Input: part model. Units: mm. Frame: model coordinates. Face numbers are marked on the shaded views. A direction names the side the tool comes from. Give positions to 0.01 mm unless a question says otherwise; leave off trailing zeros. Write each loop counter-clockwise with the first axis right and the second up, starting at its lowest first coordinate (ties: lowest second). Pieces come first, ordered by that corner, then holes. Notation, with made-up numbers: (-35, -23.75) - (5, -23.75) arc R20 ccw to (5, -0.75) - close; hole circle Ø4 at (17.5, 79). An arc over 180 degrees is marked (long way). Answer as CSV lines item,"result".
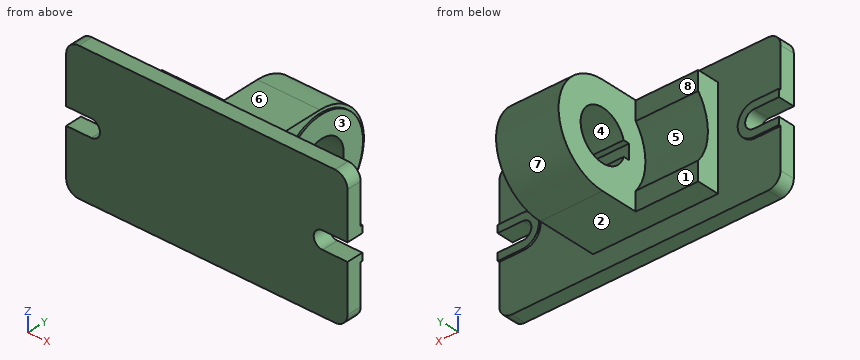
```python
from build123d import *

# Parameters (mm, degrees)
EXTRUDE_1_DEPTH     = 6
EXTRUDE_2_DEPTH     = 1.5
EXTRUDE_START       = -100
EXTRUDE_3_DEPTH     = 25
SKETCH_4_R          = 37.5
EXTRUDE_4_DEPTH     = 1.5
SKETCH_5_R          = 20
SKETCH_5_W          = 12
SKETCH_5_H          = 8
CUT_EXTRUDE_1_DEPTH = 187.58309141
SKETCH_6_W          = 50
SKETCH_6_H          = 80
EXTRUDE_5_DEPTH     = 1.5
SKETCH_7_W          = 15
SKETCH_7_H          = 16.5
EXTRUDE_6_DEPTH     = 50


with BuildPart() as part:
    # 草图1 → 凸台-拉伸1 (new, symmetric)
    with BuildSketch(Plane(origin=(0, 0, 0), x_dir=(1, 0, 0), z_dir=(0, 1, 0))):
        with BuildLine():
            ThreePointArc((-112.5, -45), (-109.571067812, -52.071067812), (-102.5, -55))
            Line((-102.5, -55), (102.5, -55))
            ThreePointArc((102.5, -55), (109.571067812, -52.071067812), (112.5, -45))
            Line((112.5, -45), (112.5, -7))
            Line((112.5, -7), (92.5, -7))
            ThreePointArc((92.5, -7), (85.5, 0), (92.5, 7))
            Line((92.5, 7), (112.5, 7))
            Line((112.5, 7), (112.5, 45))
            ThreePointArc((112.5, 45), (109.571067812, 52.071067812), (102.5, 55))
            Line((102.5, 55), (-102.5, 55))
            ThreePointArc((-102.5, 55), (-109.571067812, 52.071067812), (-112.5, 45))
            Line((-112.5, 45), (-112.5, 7))
            Line((-112.5, 7), (-92.5, 7))
            ThreePointArc((-92.5, 7), (-85.5, 0), (-92.5, -7))
            Line((-92.5, -7), (-112.5, -7))
            Line((-112.5, -7), (-112.5, -45))
        make_face()
    extrude(amount=EXTRUDE_1_DEPTH, both=True)

    # 草图2 → 凸台-拉伸2 (add, symmetric)
    with BuildSketch(Plane(origin=(0, 6, 0), x_dir=(1, 0, 0), z_dir=(0, 1, 0))):
        with BuildLine():
            Line((-92.5, 13), (-112.5, 13))
            Line((-112.5, 13), (-112.5, 7))
            Line((-112.5, 7), (-92.5, 7))
            ThreePointArc((-92.5, 7), (-85.5, 0), (-92.5, -7))
            Line((-92.5, -7), (-112.5, -7))
            Line((-112.5, -7), (-112.5, -13))
            Line((-112.5, -13), (-92.5, -13))
            ThreePointArc((-92.5, -13), (-79.5, 0), (-92.5, 13))
        make_face()
        with BuildLine():
            Line((112.5, 7), (112.5, 13))
            Line((112.5, 13), (92.5, 13))
            ThreePointArc((92.5, 13), (79.5, 0), (92.5, -13))
            Line((92.5, -13), (112.5, -13))
            Line((112.5, -13), (112.5, -7))
            Line((112.5, -7), (92.5, -7))
            ThreePointArc((92.5, -7), (85.5, 0), (92.5, 7))
            Line((92.5, 7), (112.5, 7))
        make_face()
    extrude(amount=EXTRUDE_2_DEPTH, both=True)

    # 草图3 → 凸台-拉伸3 (add, symmetric)
    with BuildSketch(Plane(origin=(112.5, 0, 0), x_dir=(0, 0, -1), z_dir=(1, 0, 0)).offset(EXTRUDE_START)):
        with BuildLine():
            Line((-40, 6), (40, 6))
            Line((40, 6), (40, 54))
            ThreePointArc((40, 54), (0, 94), (-40, 54))
            Line((-40, 54), (-40, 6))
        make_face()
    extrude(amount=EXTRUDE_3_DEPTH, both=True)

    # 草图4 → 凸台-拉伸4 (add, symmetric)
    with BuildSketch(Plane(origin=(37.5, 0, 0), x_dir=(0, 0, -1), z_dir=(1, 0, 0))):
        with Locations((0, 54)):
            Circle(SKETCH_4_R)
    extrude(amount=EXTRUDE_4_DEPTH, both=True)

    # 草图5 → 切除-拉伸1 (cut, through all)
    with BuildSketch(Plane(origin=(39, 0, 0), x_dir=(0, 0, -1), z_dir=(1, 0, 0))):
        with Locations((0, 54)):
            Circle(SKETCH_5_R)
        with Locations((0, 34)):
            Rectangle(SKETCH_5_W, SKETCH_5_H)
    extrude(amount=-CUT_EXTRUDE_1_DEPTH, mode=Mode.SUBTRACT)

    # 草图6 → 凸台-拉伸5 (add, symmetric)
    with BuildSketch(Plane(origin=(0, 6, 0), x_dir=(1, 0, 0), z_dir=(0, 1, 0))):
        with Locations((-37.5, 0)):
            Rectangle(SKETCH_6_W, SKETCH_6_H)
    extrude(amount=EXTRUDE_5_DEPTH, both=True)

    # 草图7 → 凸台-拉伸6 (add)
    with BuildSketch(Plane.ZY.offset(12.5)):
        with BuildLine():
            Line((-25, 24), (-25, 7.5))
            Line((-25, 7.5), (25, 7.5))
            Line((25, 7.5), (25, 24))
            ThreePointArc((25, 24), (0, 15.224989992), (-25, 24))
        make_face()
        with Locations((-32.5, 15.75)):
            Rectangle(SKETCH_7_W, SKETCH_7_H)
        with Locations((32.5, 15.75)):
            Rectangle(SKETCH_7_W, SKETCH_7_H)
    extrude(amount=EXTRUDE_6_DEPTH)


solid = part.part
```
Item 1: Cut plane A-A on z = 0. Return the cut outline in (x, y).
The answers:
outline,"(-85.5, -6) - (85.5, -6) - (85.5, 7.5) - (79.5, 7.5) - (79.5, 6) - (37.5, 6) - (37.5, 16.5) - (39, 16.5) - (39, 30) - (-12.5, 30) - (-12.5, 15.22) - (-62.5, 15.22) - (-62.5, 6) - (-79.5, 6) - (-79.5, 7.5) - (-85.5, 7.5) - close; (-12.5, 74) - (39, 74) - (39, 91.5) - (37.5, 91.5) - (37.5, 94) - (-12.5, 94) - close"
Item 2: Ray query, line 1 (Z direction, x = 26, y = 54); line 2 (Y direction, x = 44, z = 16); line 3 (X direction, y = 19, z = 16). Return the intervals inside material, ascending. Write a range as from..to.
The answers:
line 1,"-40..-20, 20..40"
line 2,"-6..6"
line 3,"-12.5..37.5"
Item 3: Mould query, pull axis Z, two halves, no side actions, for the marked faces 5, 6, 7 and 8. Classes: +Z half, -Z half, draft (parallel to the pull), parting line (faces both ways), or undercut.
The answers:
face 5,"undercut"
face 6,"+Z half"
face 7,"parting line"
face 8,"draft"
Item 4: Contact query for flat-ended pins moving along their axis: pin 1 (3 mm diameter, centred on y = 73.5, z = 36.5, fed in from +X); pin 2 (4.5 mm diameter, centred on x = -41, z = 36, fed in from +Y); pin 3 (2 mm diameter, centred on y = 30, z = 14, fed in from +X); pin 4 (24 mm diameter, centred on y = 54, z = 0, fed in from -X). Output: stop coordinate, or through.
The answers:
pin 1,"x = 37.5"
pin 2,"y = 24"
pin 3,"x = 39"
pin 4,"through"
Item 5: Cut plane C-C on x = 17. Return the cut outline in (y, z).
The answers:
outline,"(-6, -55) - (6, -55) - (6, -40) - (54, -40) arc R40 ccw to (54, 40) - (6, 40) - (6, 55) - (-6, 55) - close; hole (30, -6) - (34.92, -6) arc R20 ccw (long way) to (34.92, 6) - (30, 6) - close"
Item 6: Cut plane D-D on z = -35. Return the cut outline in (x, y).
The answers:
outline,"(-112.5, -6) - (112.5, -6) - (112.5, 6) - (37.5, 6) - (37.5, 40.54) - (39, 40.54) - (39, 67.46) - (37.5, 67.46) - (37.5, 73.36) - (-12.5, 73.36) - (-12.5, 24) - (-62.5, 24) - (-62.5, 6) - (-112.5, 6) - close"
Item 7: Cut plane B-B on x = -51. Return the cut outline in (y, z).
The answers:
outline,"(-6, -55) - (6, -55) - (6, -40) - (24, -40) - (24, -25) arc R40 cw to (24, 25) - (24, 40) - (6, 40) - (6, 55) - (-6, 55) - close"
Item 8: Reachability of the marked faces 1, 2, 3 and 4 from +Z, -Z, +X, -X, +Y, -Y: full face, straight path, thin tool, end or side. Return the list, or none.
The answers:
face 1,"+Z, -Z, -X, +Y"
face 2,"-Z, +X, -X, +Y"
face 3,"+Z, -Z, +X, +Y"
face 4,"+X, -X"
